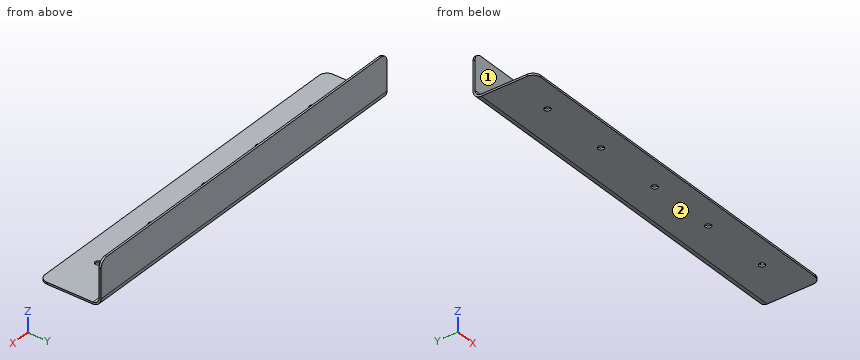
```python
from build123d import *

# Parameters (mm, degrees)
SKETCH1_W                    = 304.8
SKETCH1_H                    = 1.5875
BASE_FLANGE1_DEPTH           = 50.8
EDGE_FLANGE1_STRIP_W         = 16.51
EDGE_FLANGE1_STRIP_H         = 1.5875
EDGE_FLANGE1_STRIP_CUT_DEPTH = 304.8
EDGE_FLANGE1_DEPTH           = 304.8
SKETCH10_R                   = 2.38125
CUT_EXTRUDE1_DEPTH           = 165.439625502
FILLET1_R                    = 6.35


# Sheet-metal steps are written as plain solids
with BuildPart() as part:
    # Sketch1 → Base-Flange1 (new body)
    with BuildSketch(Plane(origin=(0, 0, 0), x_dir=(1, 0, 0), z_dir=(0, 1, 0))):
        with Locations((0, -0.79375)):
            Rectangle(SKETCH1_W, SKETCH1_H)
    extrude(amount=BASE_FLANGE1_DEPTH)

    # Edge-Flange1 strip (across the edge) → Edge-Flange1 strip cut (cut)
    with BuildSketch(Plane(origin=(152.4, 50.8, 1.5875), x_dir=(0, -1, 0), z_dir=(-1, 0, 0))):
        with Locations((-1.5875, -0.79375)):
            Rectangle(EDGE_FLANGE1_STRIP_W, EDGE_FLANGE1_STRIP_H)
    extrude(amount=EDGE_FLANGE1_STRIP_CUT_DEPTH, mode=Mode.SUBTRACT)

    # Edge-Flange1 section (across the edge) → Edge-Flange1 (add)
    with BuildSketch(Plane(origin=(152.4, 50.8, 1.5875), x_dir=(0, -1, 0), z_dir=(-1, 0, 0))):
        with BuildLine():
            Line((0, 5.08), (0, 35.1282))
            Line((0, 35.1282), (1.5875, 35.1282))
            Line((1.5875, 35.1282), (1.5875, 5.08))
            ThreePointArc((1.5875, 5.08), (3.075397552, 1.487897552), (6.6675, 0))
            Line((6.6675, 0), (6.6675, -1.5875))
            ThreePointArc((6.6675, -1.5875), (1.952865536, 0.365365536), (0, 5.08))
        make_face()
    extrude(amount=EDGE_FLANGE1_DEPTH)

    # Sketch10 → Cut-Extrude1 (cut, through all)
    with BuildSketch(Plane.XY.offset(1.5875)):
        with Locations((-114.3, 19.05)):
            Circle(SKETCH10_R)
        with Locations((114.3, 19.05)):
            Circle(SKETCH10_R)
        with Locations((0, 19.05)):
            Circle(SKETCH10_R)
        with Locations((57.15, 19.05)):
            Circle(SKETCH10_R)
        with Locations((-57.15, 19.05)):
            Circle(SKETCH10_R)
    extrude(amount=-CUT_EXTRUDE1_DEPTH, mode=Mode.SUBTRACT)

    # Fillet1
    fillet1_edges = [part.edges().sort_by_distance(p)[0] for p in [
        (152.4, 50.00625, 36.7157),
        (-152.4, 50.00625, 36.7157),
        (-152.4, 0, 0.79375),
        (152.4, 0, 0.79375),
    ]]
    fillet(fillet1_edges, radius=FILLET1_R)


solid = part.part
```
Here's how the part is built. I have some questions about the finished solid (model axes, mm). Face numbers are marked on the shaded views. A direction names the side the tool comes from. Round coordinates to 2 decimals unless told otherwise and drop trailing zeros. Order: outer loops, then holes, each group sorted by start corner. A loop starts at its lowest first (then second) coordinate and runs counter-clockwise, first axis right, second up. Notation, with made-up numbers: M -28,-3.75 L 26,-3.75 A26 cw 26,20.25 Z; hole C 35,73.5 d7. An arc over 180 degrees is marked long. Use CSV: the item, a comma, the result in double quotes.
1) I'm going to push flat-ended pins straight in: P1, Ø15, axis at x = 15.5, z = 27.5, coming from the -Y side; P2, Ø10, axis at x = -39, y = 15.5, coming from the -Z side; P3, Ø5, axis at x = -32, y = 6, coming from the +Z side. Where does each tip first touch, or does it pass through?
Taken from the geometry:
P1,"y = 49.21"
P2,"z = 0"
P3,"z = 1.59"
2) I want a section at B-B (y = 33). List the corners of the cut face in (x, z) for me, then the cut area to 3 significant figures.
Taken from the geometry:
outline,"M -152.4,0 L 152.4,0 L 152.4,1.59 L -152.4,1.59 Z"
area,"484 mm^2"
3) I want a section at C-C (z = 26.5). List the corners of the cut face in (x, y) for me.
Taken from the geometry:
outline,"M -152.4,49.21 L 152.4,49.21 L 152.4,50.8 L -152.4,50.8 Z"
4) I need wall thicknesses on line 1 along Y through (x, z) = (105, 21); line 2 along Y through (x, z) = (114.3, 1); line 3 along Z through (x, y) = (101, 9). Which ranges of each line are inside material? Lowest first, please. Write a range as [from, to].
Taken from the geometry:
line 1,"[49.21, 50.8]"
line 2,"[0, 16.67], [21.43, 47.64]"
line 3,"[0, 1.59]"
5) On a 3-axis mill with a long thin cutter (end or side, diameter ignored), from which of +Z, -Z, +X, -X, +Y, -Y can I reach the whole of each face in a straight line? I mean the marked faces 1 and 2. Say none if no direction works.
Taken from the geometry:
face 1,"+Z, +X, -X, -Y"
face 2,"-Z, +X, -X, +Y, -Y"
6) I want a section at A-A (x = 82.5). List the corners of the cut face in (y, z) for me (1 decimal).
Taken from the geometry:
outline,"M 0,0 L 44.1,0 A6.7 ccw 50.8,6.7 L 50.8,36.7 L 49.2,36.7 L 49.2,6.7 A5.1 cw 44.1,1.6 L 0,1.6 Z"
